```python
from build123d import *

# Parameters (mm, degrees)
ESTRUSIONE_ESTRUSIONE1_DEPTH = 30
SCHIZZO6_W                   = 26
SCHIZZO6_H                   = 19
TAGLIO_ESTRUSIONE2_DEPTH     = 7
TAGLIO_ESTRUSIONE3_DEPTH     = 3
TAGLIO_ESTRUSIONE3_DRAFT     = 30
FORO_10_0_10_1_D             = 10
FORO_4_0_4_1_D               = 4
RACCORDO1_R                  = 5
RACCORDO2_R                  = 6
RACCORDO3_R                  = 2
SMUSSO1_SIZE                 = 5


with BuildPart() as part:
    # Schizzo2 → Estrusione-Estrusione1 (new, symmetric)
    with BuildSketch(Plane(origin=(0, 0, 0), x_dir=(0, 0, -1), z_dir=(1, 0, 0))):
        Polygon((0, 44), (12, 44), (12, 11), (37, 11), (37, 0), (0, 0), align=None)
    extrude(amount=ESTRUSIONE_ESTRUSIONE1_DEPTH, both=True)

    # Schizzo6 → Taglio-Estrusione2 (cut)
    with BuildSketch(Plane(origin=(0, 11, 0), x_dir=(1, 0, 0), z_dir=(0, 1, 0))):
        with Locations((-17, 27.5)):
            Rectangle(SCHIZZO6_W, SCHIZZO6_H)
        with Locations((17, 27.5)):
            Rectangle(SCHIZZO6_W, SCHIZZO6_H)
    extrude(amount=-TAGLIO_ESTRUSIONE2_DEPTH, mode=Mode.SUBTRACT)


with BuildPart() as taglio_estrusione3_tool:
    # Schizzo7 → Taglio-Estrusione3 (with draft: the straight prism first)
    with BuildSketch(Plane(origin=(0, 0, -12), x_dir=(-1, 0, 0), z_dir=(0, 0, -1))):
        with BuildLine():
            Line((9.999988724, 44), (-10.000011276, 44))
            Line((-10.000011276, 44), (-10, 27.499993166))
            ThreePointArc((-10, 27.499993166), (6.834e-06, 17.5), (10, 27.500006834))
            Line((10, 27.500006834), (9.999988724, 44))
        make_face()
    extrude(amount=-TAGLIO_ESTRUSIONE3_DEPTH)
    # Taglio-Estrusione3: the draft: its side faces are tilted about the plane it starts from
    taglio_estrusione3_sides = [taglio_estrusione3_tool.faces().sort_by_distance(p)[0] for p in [
        (-9.999994362, 35.750003417, -10.5),
        (1.1276e-05, 44, -10.5),
        (10.000005638, 35.749996583, -10.5),
        (-6.834e-06, 17.5, -10.5),
    ]]
    draft(taglio_estrusione3_sides, Plane(origin=(0, 0, -12), x_dir=(-1, 0, 0), z_dir=(0, 0, -1)), TAGLIO_ESTRUSIONE3_DRAFT)


with BuildPart() as part_1:
    add(part.part)

    # Taglio-Estrusione3: cut by taglio_estrusione3_tool
    add(taglio_estrusione3_tool.part, mode=Mode.SUBTRACT)

    # Foro Ø10.0 (10)-1 (through all)
    with Locations(Plane(origin=(0, 0, -9), x_dir=(-1, 0, 0), z_dir=(0, 0, -1))):
        with Locations((-7.048e-06, 27.5)):
            Hole(FORO_10_0_10_1_D / 2)

    # Foro Ø4.0 (4)-1 (through all)
    with Locations(Plane(origin=(0, 11, 0), x_dir=(1, 0, 0), z_dir=(0, 1, 0))):
        with Locations((0, 31), (-24, 15), (24, 15)):
            Hole(FORO_4_0_4_1_D / 2)

    # Raccordo1
    raccordo1_edges = [part_1.edges().sort_by_distance(p)[0] for p in [
        (30, 44, -6),
        (-30, 44, -6),
    ]]
    fillet(raccordo1_edges, radius=RACCORDO1_R)

    # Raccordo2
    raccordo2_edges = [part_1.edges().sort_by_distance(p)[0] for p in [
        (-4, 7.5, -18),
        (4, 7.5, -18),
    ]]
    fillet(raccordo2_edges, radius=RACCORDO2_R)

    # Raccordo3
    raccordo3_edges = [part_1.edges().sort_by_distance(p)[0] for p in [
        (-30, 7.5, -18),
        (-4, 7.5, -37),
        (4, 7.5, -37),
        (30, 7.5, -18),
    ]]
    fillet(raccordo3_edges, radius=RACCORDO3_R)

    # Smusso1
    smusso1_edges = [part_1.edges().sort_by_distance(p)[0] for p in [
        (30, 2, -37),
        (-30, 2, -37),
    ]]
    chamfer(smusso1_edges, length=SMUSSO1_SIZE)


solid = part_1.part
```
Input: part model. Units: mm. Frame: model coordinates. A direction names the side the tool comes from. Round coordinates to 2 decimals unless told otherwise and drop trailing zeros. Loops run counter-clockwise (first coordinate to the right, second up) from the corner with the lowest first, then second, coordinate; pieces in that order, holes last.
1) Set-up query: faces 4 (the flat face through (0, 0, -19)), 5 (the flat face through (-16, 4, -27)), 6 (the cylindrical face through (25.474, 5.423, -16.352)), 7 (the flat face through (16, 4, -27)), 8 (the flat face through (7, 20, -12)). Return all of +Z, -Z, +X, -X, +Y, -Y with unobstructed straight access to the full face (end or side cutting, diameter ignored); none if empty.
Ans:
face 4: +Z, -Z, +X, -X, -Y
face 5: -Z, -X, +Y
face 6: +Y, -Y
face 7: -Z, +X, +Y
face 8: -Z, +X, -X, +Y
2) Pin query (flat end, axial travel): pin 1 (10.5 mm diameter, centred on x = 12, z = -30, fed in from +Y); pin 2 (16.5 mm diameter, centred on x = -11, y = 31, fed in from -Z); pin 3 (1.5 mm diameter, centred on x = 9, y = 26, fed in from -Z); pin 4 (8 mm diameter, centred on x = 0, y = 27.5, fed in from +Z). Return the tip coordinate at first contact, or that it passes through.
Ans:
pin 1: stops at y = 4
pin 2: stops at z = -12
pin 3: stops at z = -9
pin 4: passes through
3) Material intervals for line 1 (X direction, y = 9, z = -15); line 2 (Z direction, x = -2.5, y = 39); line 3 (Z direction, x = -9.5, y = 19), sorted ascending.
Ans:
line 1: x = -30 to -26, -22 to 22, 26 to 30
line 2: z = -9 to 0
line 3: z = -12 to 0
4) Section query A-A on x = 0. Return the cut outline in (y, z).
Ans:
outline: (0, -37) - (11, -37) - (11, -33) - (0, -33) - close; (0, -29) - (11, -29) - (11, -12) - (17.5, -12) - (15.77, -9) - (22.5, -9) - (22.5, 0) - (0, 0) - close; (32.5, -9) - (44, -9) - (44, 0) - (32.5, 0) - close
5) Pull-direction query (X, two-part tool) for faces 1 (the cylindrical face through (28, 43, -6)), 2 (the flat face through (0, 44, -6)), 3 (the cylindrical face through (-22.526, 5.423, -16.352)); classes: released by +X, released by -X, zero draft, split by the parting line, or undercut.
Ans:
face 1: released by +X
face 2: zero draft
face 3: undercut
6) Section query C-C on x = -24. Return the cut outline in (y, z), plus the area to 3 significant figures.
Ans:
outline: (0, -37) - (4, -37) - (4, -18) - (11, -18) - (11, -17) - (0, -17) - close; (0, -13) - (11, -13) - (11, -12) - (44, -12) - (44, 0) - (0, 0) - close
area: 626 mm2
7) Section query B-B on y = 29.5. Return the cut outline in (x, z), plus the area to 3 significant figures.
Ans:
outline: (-30, -12) - (-10, -12) - (-11.73, -9) - (-4.58, -9) - (-4.58, 0) - (-30, 0) - close; (4.58, -9) - (11.73, -9) - (10, -12) - (30, -12) - (30, 0) - (4.58, 0) - close
area: 572 mm2
8) Section query D-D on y = 5.5. Return the cut outline in (x, z).
Ans:
outline: (-30, -16) arc R2 ccw to (-28, -18) - (-10, -18) arc R6 cw to (-4, -24) - (-4, -35) arc R2 ccw to (-2, -37) - (2, -37) arc R2 ccw to (4, -35) - (4, -24) arc R6 cw to (10, -18) - (28, -18) arc R2 ccw to (30, -16) - (30, 0) - (-30, 0) - close; hole circle Ø4 at (-24, -15); hole circle Ø4 at (0, -31); hole circle Ø4 at (24, -15)
